CAD build for the part. Positions are in the model's coordinates, mm. Coordinates: 2 decimals unless noted, no trailing zeros. Write each loop counter-clockwise with the first axis right and the second up, starting at its lowest first coordinate (ties: lowest second). Pieces come first, ordered by that corner, then holes. Notation, with made-up numbers: (-32, 12.25) -> (-22, 12.25) arc R10 ccw to (-22, 16.25) -> close; hole circle Ø5 at (57, 42). An arc over 180 degrees is marked (long way). Answer as CSV lines item,"result". Start each with the question number.
```python
from build123d import *

# Parameters (mm, degrees)
PAD_DEPTH            = 1.8
SKETCH004_R          = 2.875
PAD001_DEPTH         = 5
SKETCH005_R          = 1
POCKET_DEPTH         = 1.801
BODY_PLACEMENT_ANGLE = 90


with BuildPart() as part:
    # Sketch → Pad (new body)
    with BuildSketch(Plane.XY):
        with BuildLine():
            ThreePointArc((5, 0), (0, 5), (-5, 0))
            Line((-5, -11.5), (-5, 0))
            Line((5, -11.5), (-5, -11.5))
            Line((5, 0), (5, -11.5))
        make_face()
    extrude(amount=PAD_DEPTH)

    # Sketch004 (on Face6 of Pad) → Pad001 (join)
    with BuildSketch(Plane.XY.offset(1.8)):
        Circle(SKETCH004_R)
    extrude(amount=PAD001_DEPTH)

    # Sketch005 (on Face5 of Pad001) → Pocket (cut, through all)
    with BuildSketch(Plane.XY.offset(1.8)):
        with Locations((-2.5, -8.910861)):
            Circle(SKETCH005_R)
        with Locations((2.5, -8.910861)):
            Circle(SKETCH005_R)
    extrude(amount=-POCKET_DEPTH, mode=Mode.SUBTRACT)


with BuildPart() as part_1:
    # Body placement: moved
    add(part.part.rotate(Axis((0, 0, 0), (0, 0, 1)), BODY_PLACEMENT_ANGLE))


solid = part_1.part
```
1. Cut at A-A (y = 2.5). Give the cut face in (x, z), then the cut area to 3 significant figures.
2. Cut at D-D (z = 1). Give the cut face in (x, y).
3. Cut at B-B (y = 0). Give the cut face in (x, z) (3 decimals).
4. Wall check: line 1 (Z direction, x = 1.25, y = 4.75); line 2 (X direction, y = -2.5, z = 1.25); line 3 (X direction, y = 3.75, z = 1.75). Give the ranges that are in metal, low to high.
5. Flat gauge pins, fed straight in: P1, Ø1.5, axis at x = 8.5, z = 2.5, coming from the -Y side; P2, Ø4, axis at y = -2.5, z = 3, coming from the -X side. Where does each tip first touch, or does it go through?
6. Cut at C-C (x = 8.5). Give the cut face in (y, z).
7. Mould opens along X. For faces 1 (the face through (7.92, -2.63, 0.91)), 2 (the face through (-2.85, -0.37, 4.26)), 3 (the face through (8.24, 1.76, 0.91)), 4 (the face through (6, 5, 1)) say: pulls with the +X half, pulls with the -X half, needs draft (parallel to the pull), parting line crosses it, or undercut.
Geometry check:
1,outline,"(-4.33, 0) -> (7.91, 0) -> (7.91, 1.8) -> (1.42, 1.8) -> (1.42, 6.8) -> (-1.42, 6.8) -> (-1.42, 1.8) -> (-4.33, 1.8) -> close; (9.91, 0) -> (11.5, 0) -> (11.5, 1.8) -> (9.91, 1.8) -> close"
1,area,"39.1 mm²"
2,outline,"(0, -5) -> (11.5, -5) -> (11.5, 5) -> (0, 5) arc R5 ccw to start; hole circle Ø2 at (8.91, -2.5); hole circle Ø2 at (8.91, 2.5)"
3,outline,"(-5, 0) -> (11.5, 0) -> (11.5, 1.8) -> (2.875, 1.8) -> (2.875, 6.8) -> (-2.875, 6.8) -> (-2.875, 1.8) -> (-5, 1.8) -> close"
4,line 1,"0 to 1.8"
4,line 2,"-4.33 to 7.91, 9.91 to 11.5"
4,line 3,"-3.31 to 11.5"
5,P1,"y = -5"
5,P2,"x = -4.92"
6,outline,"(-5, 0) -> (-3.41, 0) -> (-3.41, 1.8) -> (-5, 1.8) -> close; (-1.59, 0) -> (1.59, 0) -> (1.59, 1.8) -> (-1.59, 1.8) -> close; (3.41, 0) -> (5, 0) -> (5, 1.8) -> (3.41, 1.8) -> close"
7,face 1,"undercut"
7,face 2,"parting line crosses it"
7,face 3,"undercut"
7,face 4,"needs draft"
